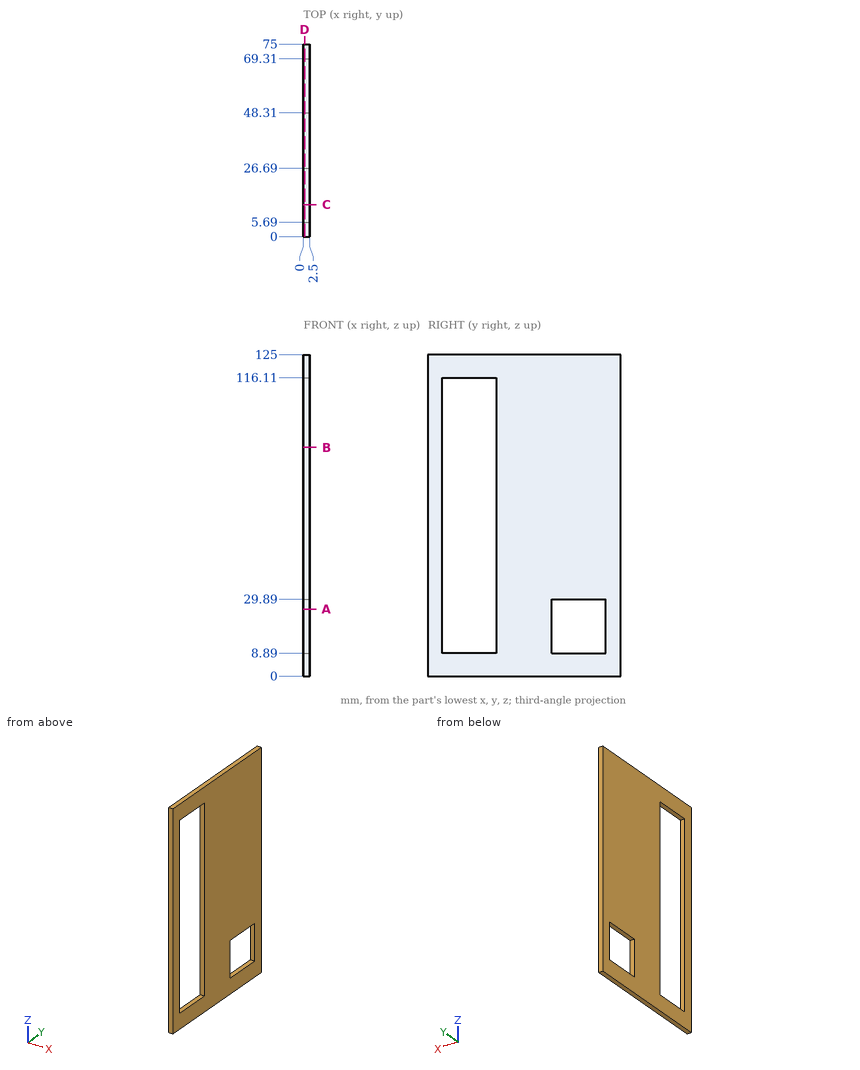
Check sheet for the drawn part. Datum: minimum x, y, z corner. Units: mm. Round coordinates to 2 decimals unless told otherwise and drop trailing zeros. Order: outer loops, then holes, each group sorted by start corner. A loop starts at its lowest first (then second) coordinate and runs counter-clockwise, first axis right, second up. Notation, with made-up numbers: (52, 68) - (89, 68) arc R15 cw to (89, 94) - close; hole circle Ø5 at (-25, 68.25). An arc over 180 degrees is marked (long way). Use a Markdown table: item, result. Add a question column.
(1) Material ranges on line 1 along Y through (x, z) = (0.5, 10); line 2 along Z through (x, y) = (2, 59.5); line 3 along Z through (x, y) = (0.45, 12.5), recorded low to high. Write a range as [from, to].
(2) Sectioned sample at B-B, the plane z = 89. Enter the section's corners in (x, y), and give its area (3 significant figures).
(3) Sectioned sample at C-C, the plane y = 12.5. Enter the section's corners in (x, z).
(4) Depth check by flat-ended pin: pin 1 (12 mm diameter, centred on y = 26.5, z = 108, fed in from +X). Enter the tip coordinate at first touch or a pass-through.
(5) Sectioned sample at D-D, the plane x = 0.5. Enter the section's corners in (y, z), and give its area (3 significant figures).
(6) Sectioned sample at A-A, the plane z = 26. Enter the section's corners in (x, y).
Answers below:
| question | item | result |
|---|---|---|
| 1 | line 1 | [0, 5.69], [26.69, 48.31], [69.31, 75] |
| 1 | line 2 | [0, 8.89], [29.89, 125] |
| 1 | line 3 | [0, 8.89], [116.11, 125] |
| 2 | outline | (0, 0) - (2.5, 0) - (2.5, 5.69) - (0, 5.69) - close; (0, 26.69) - (2.5, 26.69) - (2.5, 75) - (0, 75) - close |
| 2 | area | 135 mm² |
| 3 | outline | (0, 0) - (2.5, 0) - (2.5, 8.89) - (0, 8.89) - close; (0, 116.11) - (2.5, 116.11) - (2.5, 125) - (0, 125) - close |
| 4 | pin 1 | x = 2.5 |
| 5 | outline | (0, 0) - (75, 0) - (75, 125) - (0, 125) - close; hole (5.69, 8.89) - (26.69, 8.89) - (26.69, 116.11) - (5.69, 116.11) - close; hole (48.31, 8.89) - (69.31, 8.89) - (69.31, 29.89) - (48.31, 29.89) - close |
| 5 | area | 6,680 mm² |
| 6 | outline | (0, 0) - (2.5, 0) - (2.5, 5.69) - (0, 5.69) - close; (0, 26.69) - (2.5, 26.69) - (2.5, 48.31) - (0, 48.31) - close; (0, 69.31) - (2.5, 69.31) - (2.5, 75) - (0, 75) - close |
